from build123d import *

# Parameters (mm, degrees)
F0_W     = 10
F0_H     = 20
F1_DEPTH = 10
F2_DEPTH = 20
F3_R     = 0.5


with BuildPart() as f1:
    # F0 (on Front) → F1 (new body)
    with BuildSketch(Plane.XZ):
        Polygon((-10, 56.511319), (-10, 21.511319), (0, 21.511319), (0, 11.511319), (10, 11.511319), (10, 56.511319), align=None)
        Polygon((10, -8.488681), (0, -8.488681), (0, -18.488681), (-11.420748, -18.488681), (-11.420748, -53.488681), (10, -53.488681), align=None)
        with Locations((5, 1.511319)):
            Rectangle(F0_W, F0_H)
    extrude(amount=F1_DEPTH)

    # F0 (on Front) → F2 (join)
    with BuildSketch(Plane.XZ):
        Polygon((-10, 56.511319), (-10, 21.511319), (0, 21.511319), (0, 11.511319), (10, 11.511319), (10, 56.511319), align=None)
        Polygon((10, -8.488681), (0, -8.488681), (0, -18.488681), (-11.420748, -18.488681), (-11.420748, -53.488681), (10, -53.488681), align=None)
    extrude(amount=F2_DEPTH)

    # F3
    f3_edges = [f1.edges().sort_by_distance(p)[0] for p in [
        (-10, -20, 39.011319),
        (-5, -20, 21.511319),
        (0, -20, 16.511319),
        (5, -20, 11.511319),
        (10, -20, 34.011319),
        (0, -20, 56.511319),
        (5, -20, -8.488681),
        (0, -20, -13.488681),
        (-5.710374, -20, -18.488681),
        (-11.420748, -20, -35.988681),
        (-0.710374, -20, -53.488681),
        (10, -20, -30.988681),
        (-10, -10, 56.511319),
        (-10, -10, 21.511319),
        (-10, 0, 39.011319),
        (-11.420748, -10, -18.488681),
        (-11.420748, -10, -53.488681),
        (-11.420748, 0, -35.988681),
        (0, -10, 21.511319),
        (0, -15, 11.511319),
        (0, -10, 1.511319),
        (0, -15, -8.488681),
        (0, -10, -18.488681),
        (0, 0, 1.511319),
        (0, 0, 56.511319),
        (-5, 0, 21.511319),
        (-5.710374, 0, -18.488681),
        (-0.710374, 0, -53.488681),
        (10, 0, 1.511319),
        (10, -10, -53.488681),
        (10, -15, -8.488681),
        (10, -10, 1.511319),
        (10, -15, 11.511319),
        (10, -10, 56.511319),
    ]]
    fillet(f3_edges, radius=F3_R)


solid = f1.part
Geometry check sheet. Reference: the model listing, model coordinates, mm. A direction names the side the tool comes from. Coordinates: 2 decimals unless noted, no trailing zeros. Order: outer loops, then holes, each group sorted by start corner. A loop starts at its lowest first (then second) coordinate and runs counter-clockwise, first axis right, second up. Notation, with made-up numbers: (-38.5, -23.75) - (-28.5, -23.75) arc R25 ccw to (-28.5, 7.25) - close; hole circle Ø10 at (39, 79). An arc over 180 degrees is marked (long way). One line per item, written item: value.
(1) Sectioned sample at D-D (x = 8.25). Enter the section's corners in (y, z), and give its area (3 significant figures).
Data:
outline: (-20, -52.99) arc R0.5 ccw to (-19.5, -53.49) - (-0.5, -53.49) arc R0.5 ccw to (0, -52.99) - (0, 56.01) arc R0.5 ccw to (-0.5, 56.51) - (-19.5, 56.51) arc R0.5 ccw to (-20, 56.01) - (-20, 12.01) arc R0.5 ccw to (-19.5, 11.51) - (-10, 11.51) - (-10, -8.49) - (-19.5, -8.49) arc R0.5 ccw to (-20, -8.99) - close
area: 2,000 mm^2
(2) Sectioned sample at A-A (x = -4.5). Enter the section's corners in (y, z), and give its area (3 significant figures).
Data:
outline: (-20, -52.99) arc R0.5 ccw to (-19.5, -53.49) - (-0.5, -53.49) arc R0.5 ccw to (0, -52.99) - (0, -18.99) arc R0.5 ccw to (-0.5, -18.49) - (-19.5, -18.49) arc R0.5 ccw to (-20, -18.99) - close; (-20, 22.01) arc R0.5 ccw to (-19.5, 21.51) - (-0.5, 21.51) arc R0.5 ccw to (0, 22.01) - (0, 56.01) arc R0.5 ccw to (-0.5, 56.51) - (-19.5, 56.51) arc R0.5 ccw to (-20, 56.01) - close
area: 1,400 mm^2
(3) Sectioned sample at B-B (y = -16.5). Enter the section's corners in (x, z).
Data:
outline: (-11.42, -52.99) arc R0.5 ccw to (-10.92, -53.49) - (9.5, -53.49) arc R0.5 ccw to (10, -52.99) - (10, -8.99) arc R0.5 ccw to (9.5, -8.49) - (0.5, -8.49) arc R0.5 ccw to (0, -8.99) - (0, -17.99) arc R0.5 cw to (-0.5, -18.49) - (-10.92, -18.49) arc R0.5 ccw to (-11.42, -18.99) - close; (-10, 22.01) arc R0.5 ccw to (-9.5, 21.51) - (-0.5, 21.51) arc R0.5 cw to (0, 21.01) - (0, 12.01) arc R0.5 ccw to (0.5, 11.51) - (9.5, 11.51) arc R0.5 ccw to (10, 12.01) - (10, 56.01) arc R0.5 ccw to (9.5, 56.51) - (-9.5, 56.51) arc R0.5 ccw to (-10, 56.01) - close
(4) Access from +Z, -Z, +X, -X, +Y, -Y to the whole of each face (thin tool, end or side, straight path). Record for faces 1 (the face through (-1, -10, -53.489)), 2 (the face through (-5, -10, 21.511)), 3 (the face through (-10, -10, 39)), 4 (the face through (5, -15, 11.511)), 5 (the face through (-1, -20, -31)).
Data:
face 1: -Z, +X, -X, +Y, -Y
face 2: -X, +Y, -Y
face 3: +Z, -X, +Y, -Y
face 4: +X, -X, -Y
face 5: +Z, -Z, +X, -X, -Y
(5) Release check for a two-part mould opening along Z. For faces 6 (the face through (5, -10, 2)), 7 (the face through (10, -8, 1)), 8 (the face through (0, -10, 56.511)) record: +Z half, -Z half, draft (parallel to the pull), parting line (faces both ways), or undercut.
Data:
face 6: undercut
face 7: draft
face 8: +Z half
(6) Thickness scan on probe 1 along Z at (x, y) = (-6.25, -9.75); probe 2 along Z at (x, y) = (7.5, -11.25); probe 3 along Y at (x, z) = (6.5, 2). Record the ranges inside material, lowest first. Write a range as from..to.
Data:
probe 1: z = -53.49..-18.49, 21.51..56.51
probe 2: z = -53.49..-8.49, 11.51..56.51
probe 3: y = -10..0
(7) Sectioned sample at C-C (z = -16.5). Enter the section's corners in (x, y), and give its area (3 significant figures).
Data:
outline: (0, -19.5) arc R0.5 ccw to (0.5, -20) - (9.5, -20) arc R0.5 ccw to (10, -19.5) - (10, -0.5) arc R0.5 ccw to (9.5, 0) - (0.5, 0) arc R0.5 ccw to (0, -0.5) - close
area: 200 mm^2
(8) Depth check by flat-ended pin: pin 1 Ø10 at (x, z) = (6, -0.5) entering from -Y; pin 2 Ø3 at (y, z) = (-5.5, 43) entering from -X. Enter the tip coordinate at first touch or a pass-through.
Data:
pin 1: stops at y = -10
pin 2: stops at x = -10
